Geometry: final body of the model. Coordinates: model frame, mm. A direction names the side the tool comes from. Give positions to 0.01 mm unless a question says otherwise; leave off trailing zeros. Write each loop counter-clockwise with the first axis right and the second up, starting at its lowest first coordinate (ties: lowest second). Pieces come first, ordered by that corner, then holes. Notation, with made-up numbers: (-37, 5.25) -> (20, 5.25) arc R19 cw to (20, 39.25) -> close; hole circle Ø5 at (0.5, -25). An arc over 180 degrees is marked (long way). Use CSV: the item, a comma, the result in double quotes. Start each with the question number.
1) Draft query along Y for faces 1 (the face through (-3.755, -35.908, 11.923)), 2 (the face through (8, -33.1, 0)). Return one class per face: pulls with the +Y half, pulls with the -Y half, needs draft (parallel to the pull), parting line crosses it, or undercut.
2) Material intervals for line 1 (Y direction, x = 2, z = 5.5); line 2 (X direction, y = -2.5, z = -7); line 3 (Z direction, x = -4.5, y = -3.5), sorted ascending. Write a range as [from, to].
3) Section C-C (y = -28). Output: boundary loops of the cut face in (x, z), plus the area to 3 significant figures.
4) Contact query for flat-ended pins moving along their axis: P1, Ø3, axis at x = -7.5, y = -31, coming from the -Z side; P2, Ø1, axis at y = -35, z = -7.5, coming from the +X side; P3, Ø5, axis at y = -15, z = 3.5, coming from the +X side. Output: stop coordinate, or through.
5) Set-up query: faces 3 (the face through (-3.755, -29.108, 11.923)), 4 (the face through (-3.04, -23.98, -3.32)). Return all of +Z, -Z, +X, -X, +Y, -Y with unobstructed straight access to the full face (end or side cutting, diameter ignored); none if empty.
6) Section A-A (z = -10). Count the separate pieces of the cut face and the enclosed holes in it, plus the area to 3 significant figures.
```python
from build123d import *

# Parameters (mm, degrees)
SKETCH2_W           = 8
SKETCH2_H           = 2.2
LPATTERN1_COUNT     = 9
LPATTERN1_PITCH     = 3.4
BOSS_EXTRUDE1_REACH = 55.127
SKETCH3_R           = 7.5
SKETCH4_R           = 6
BOSS_EXTRUDE2_DEPTH = 2.2


with BuildPart() as part:
    # Sketch1 → Revolve1 (revolve)
    with BuildSketch(Plane.XY, mode=Mode.PRIVATE) as revolve1_sk:
        Polygon((0, 0), (8, 0), (8, -3.7), (6, -3.7), (6, -9.3), (8, -9.3), (8, -12.3), (4.5, -12.3), (4.5, -14.6), (8, -14.6), (8, -16), (4.5, -16), (4.5, -18.3), (12.5, -18.3), (12.5, -50.1), (0, -50.1), align=None)
    revolve(revolve1_sk.sketch.rotate(Axis((0, 0, 0), (0, -1, 0)), 90), axis=Axis((0, 0, 0), (0, -1, 0)))

    # Sketch2 → Cut-Revolve3 (revolve, cut)
    with BuildSketch(Plane.XY, mode=Mode.PRIVATE) as cut_revolve3_sk:
        with Locations((8.5, -47.8)):
            Rectangle(SKETCH2_W, SKETCH2_H)
    cut_revolve3 = revolve(cut_revolve3_sk.sketch.rotate(Axis((0, 0, 0), (0, -1, 0)), 90), axis=Axis((0, 0, 0), (0, -1, 0)), mode=Mode.SUBTRACT)

    # LPattern1: Cut-Revolve3 ×9
    with Locations(*[(0, i * LPATTERN1_PITCH, 0) for i in range(1, LPATTERN1_COUNT)]):
        add(cut_revolve3, mode=Mode.SUBTRACT)

    # Boss-Extrude1: up to this face of the body (flat: up to its plane)
    boss_extrude1_end = Plane(part.part.faces().sort_by_distance((0, -31.9, -4.853553391))[0])
    # Sketch3 → Boss-Extrude1 (add, up to the picked face)
    with BuildSketch(Plane.XZ.offset(50.1), mode=Mode.PRIVATE) as boss_extrude1_sk1:
        with Locations(Location((0, 0, 0), (0, 0, 270))):
            Circle(SKETCH3_R)
    boss_extrude1_tool1 = split(extrude(boss_extrude1_sk1.sketch, amount=-BOSS_EXTRUDE1_REACH, mode=Mode.PRIVATE), bisect_by=boss_extrude1_end, keep=Keep.BOTH, mode=Mode.PRIVATE)
    add(boss_extrude1_tool1.solids().sort_by(Axis((0, -50.1, 0), (0, 1, 0)))[0])

    # Sketch4 → Boss-Extrude2 (add)
    with BuildSketch(Plane(origin=(0, -31.9, 0), x_dir=(1, 0, 0), z_dir=(0, 1, 0))):
        with Locations(Location((0, 0, 0), (0, 0, 270))):
            Circle(SKETCH4_R)
    extrude(amount=BOSS_EXTRUDE2_DEPTH)


solid = part.part
```
Answers follow:
1,face 1,"needs draft"
1,face 2,"undercut"
2,line 1,"y = [-50.1, -28.5], [-26.3, -25.1], [-22.9, -21.7], [-19.5, -18.3], [-16, -14.6], [-12.3, 0]"
2,line 2,"x = [-3.87, 3.87]"
2,line 3,"z = [-6.61, 6.61]"
3,outline,"circle Ø9 at (0, 0)"
3,area,"63.6 mm^2"
4,P1,"stops at z = -10.8"
4,P2,"stops at x = 10.29"
4,P3,"stops at x = 7.94"
5,face 3,"+Y, -Y"
5,face 4,"none"
6,separate pieces,"10"
6,enclosed holes,"0"
6,area,"180 mm^2"
